Part print with two shaded views. Sizes in mm from the minimum x, y, z corner. Give positions to 0.01 mm unless a question says otherwise; leave off trailing zeros. Write each loop counter-clockwise with the first axis right and the second up, starting at its lowest first coordinate (ties: lowest second). Pieces come first, ordered by that corner, then holes. Notation, with made-up numbers: (-23, 25) -> (30, 25) arc R20 ccw to (30, 32) -> close; hole circle Ø10 at (-28, -13). An arc over 180 degrees is marked (long way). Answer as a JSON object with one key per item and string values.
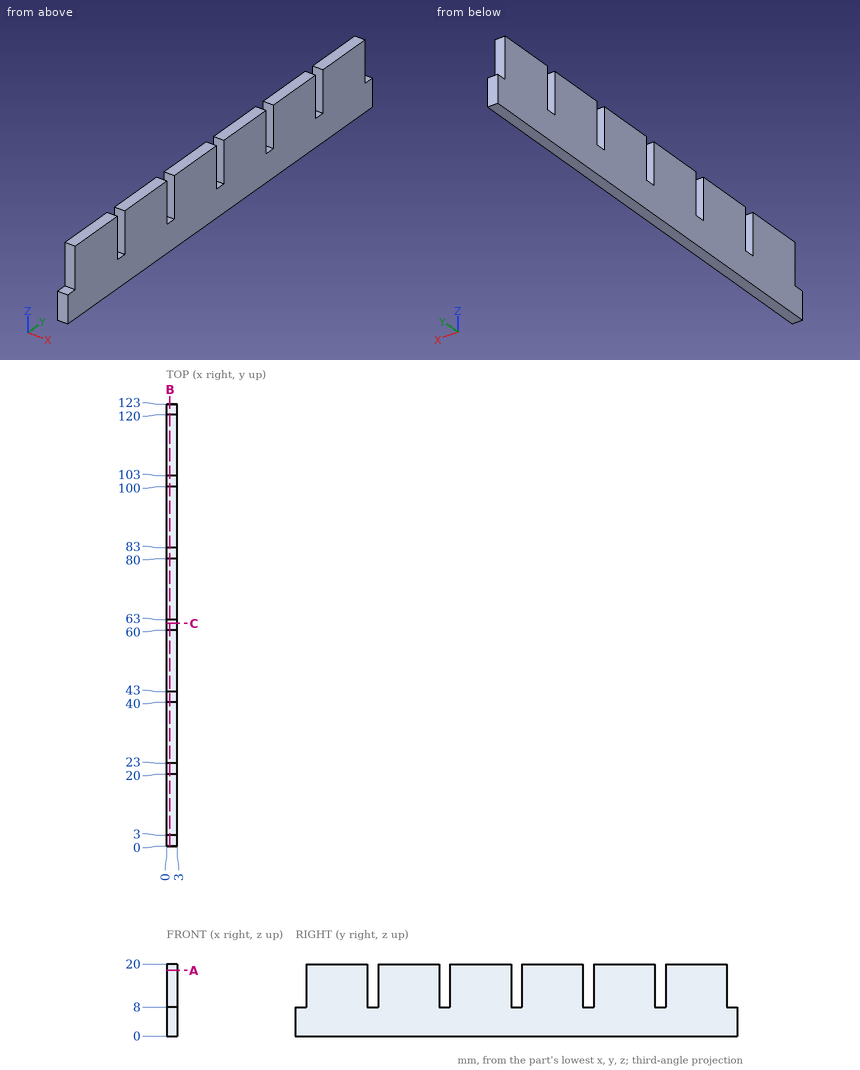
1) Slice it at A-A (z = 18.25). List the corners of the cut face in (x, y), then the cut area to 3 significant figures.
Model answer:
{"outline": "(0, 3) -> (3, 3) -> (3, 20) -> (0, 20) -> close; (0, 23) -> (3, 23) -> (3, 40) -> (0, 40) -> close; (0, 43) -> (3, 43) -> (3, 60) -> (0, 60) -> close; (0, 63) -> (3, 63) -> (3, 80) -> (0, 80) -> close; (0, 83) -> (3, 83) -> (3, 100) -> (0, 100) -> close; (0, 103) -> (3, 103) -> (3, 120) -> (0, 120) -> close", "area": "306 mm2"}
2) Slice it at B-B (x = 0.9). List the corners of the cut face in (y, z).
Model answer:
{"outline": "(0, 0) -> (123, 0) -> (123, 8) -> (120, 8) -> (120, 20) -> (103, 20) -> (103, 8) -> (100, 8) -> (100, 20) -> (83, 20) -> (83, 8) -> (80, 8) -> (80, 20) -> (63, 20) -> (63, 8) -> (60, 8) -> (60, 20) -> (43, 20) -> (43, 8) -> (40, 8) -> (40, 20) -> (23, 20) -> (23, 8) -> (20, 8) -> (20, 20) -> (3, 20) -> (3, 8) -> (0, 8) -> close"}
3) Pin check, flat tips, straight feed: pin 1 (0.9 mm diameter, centred on x = 1.5, z = 13, fed in from -Y); pin 2 (1.5 mm diameter, centred on x = 1, y = 101.5, fed in from +Z); pin 3 (1.5 mm diameter, centred on x = 1, z = 14.5, fed in from +Y). Stop position of each tip, or through.
Model answer:
{"pin 1": "stops at y = 3", "pin 2": "stops at z = 8", "pin 3": "stops at y = 120"}
4) Wall check: probe 1 along Y at (x, z) = (0.8, 14.25); probe 2 along Z at (x, y) = (2.2, 41). Give the ranges that are in metal, low to high.
Model answer:
{"probe 1": "y = 3 to 20, 23 to 40, 43 to 60, 63 to 80, 83 to 100, 103 to 120", "probe 2": "z = 0 to 8"}
5) Slice it at C-C (y = 62). List the corners of the cut face in (x, z), then the cut area to 3 significant figures.
Model answer:
{"outline": "(0, 0) -> (3, 0) -> (3, 8) -> (0, 8) -> close", "area": "24.0 mm2"}
